For this review, take the finished solid that the model builds, in its own axes (mm). Face numbers are marked on the shaded views. A direction names the side the tool comes from. Give positions to 0.01 mm unless a question says otherwise; leave off trailing zeros. Write each loop counter-clockwise with the first axis right and the second up, starting at its lowest first coordinate (ties: lowest second). Pieces come first, ordered by that corner, then holes. Notation, with made-up numbers: M 59.25,-25.5 L 112.25,-25.5 A23 cw 112.25,8.5 Z; hole C 45,-13 d7. An arc over 180 degrees is marked long. Write item = value, one per line.
```python
from build123d import *

# Parameters (mm, degrees)
F1_DEPTH = 8
F2_R     = 3
F3_DEPTH = 8
F4_R     = 4
F5_DEPTH = 8
F6_W     = 9
F6_H     = 2
F7_DEPTH = 3


with BuildPart() as f1:
    # F0 (on Top) → F1 (new body)
    with BuildSketch(Plane.XY):
        with BuildLine():
            Line((7, 20), (-7, 20))
            ThreePointArc((-7, 20), (-9.12132, 19.12132), (-10, 17))
            Line((-10, 17), (-10, -17))
            ThreePointArc((-10, -17), (-9.12132, -19.12132), (-7, -20))
            Line((-7, -20), (7, -20))
            ThreePointArc((7, -20), (9.12132, -19.12132), (10, -17))
            Line((10, -17), (10, 17))
            ThreePointArc((10, 17), (9.12132, 19.12132), (7, 20))
        make_face()
    extrude(amount=F1_DEPTH)

    # F2 (on face) → F3 (cut, through all)
    with BuildSketch(Plane.XY.offset(8)):
        with Locations((0, 12)):
            Circle(F2_R)
        with Locations((0, -12)):
            Circle(F2_R)
    extrude(amount=-F3_DEPTH, mode=Mode.SUBTRACT)

    # F4 (on face) → F5 (cut, through all)
    with BuildSketch(Plane.XY.offset(8)):
        Circle(F4_R)
    extrude(amount=-F5_DEPTH, mode=Mode.SUBTRACT)

    # F6 (on face) → F7 (join)
    with BuildSketch(Plane.XY.offset(8)):
        with Locations((0, -6.5)):
            Rectangle(F6_W, F6_H)
        with Locations((0, 6.5)):
            Rectangle(F6_W, F6_H)
    extrude(amount=F7_DEPTH)


solid = f1.part
```
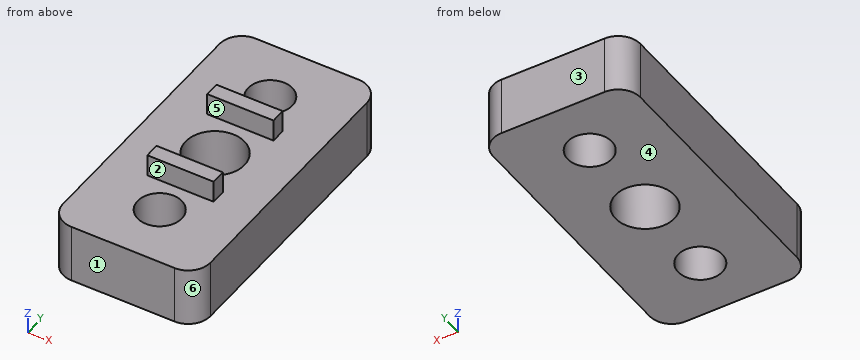
1. The part is to be moulded in two halves that separate along Y. For the marked faces 3, 4, 5 and 6, say which applies: +Y half, -Y half, draft (parallel to the pull), parting line (faces both ways), or undercut.
Responses:
face_3 = +Y half
face_4 = draft
face_5 = undercut
face_6 = -Y half
2. For line 1 along Y through (x, z) = (0, 5); line 2 along Y through (x, z) = (2.5, 4.5); line 3 along Z through (x, y) = (7, -4), list the stretches that pass through material, from the lowest coordinate up. Write a range as from..to.
Responses:
line_1 = -20..-15, -9..-4, 4..9, 15..20
line_2 = -20..-13.66, -10.34..-3.12, 3.12..10.34, 13.66..20
line_3 = 0..8
3. Machinability: for the marked faces 1 and 2, which of the approach directions +Z, -Z, +X, -X, +Y, -Y give a long, thin tool a straight path to every point of the face, cutting with its end or side? Answer none if there is none.
Responses:
face_1 = +Z, -Z, +X, -X, -Y
face_2 = +Z, +X, -X, -Y
4. Insertion check: P1, Ø1.6, axis at y = -6.5, z = 9, coming from the -X side; P2, Ø2.5, axis at x = -1.5, z = 10, coming from the -Y side; P3, Ø5, axis at x = 7, y = 1.5, coming from the +Z side. Each pin has a flat end and moves straight along its axis. Give the tip position at first contact, or say it passes through.
Responses:
P1 = -4.5
P2 = -7.5
P3 = 8
5. We need section C-C, the plane x = 0. Write out the cut boundary in (y, z).
Responses:
outline = M -20,0 L -15,0 L -15,8 L -20,8 Z; M -9,0 L -4,0 L -4,8 L -5.5,8 L -5.5,11 L -7.5,11 L -7.5,8 L -9,8 Z; M 4,0 L 9,0 L 9,8 L 7.5,8 L 7.5,11 L 5.5,11 L 5.5,8 L 4,8 Z; M 15,0 L 20,0 L 20,8 L 15,8 Z
6. We need section D-D, the plane z = 4. Write out the cut boundary in (x, y).
Responses:
outline = M -10,-17 A3 ccw -7,-20 L 7,-20 A3 ccw 10,-17 L 10,17 A3 ccw 7,20 L -7,20 A3 ccw -10,17 Z; hole C 0,0 d8; hole C 0,-12 d6; hole C 0,12 d6
7. We need section B-B, the plane z = 8.5. Write out the cut boundary in (x, y).
Responses:
outline = M -4.5,-7.5 L 4.5,-7.5 L 4.5,-5.5 L -4.5,-5.5 Z; M -4.5,5.5 L 4.5,5.5 L 4.5,7.5 L -4.5,7.5 Z
8. We need section A-A, the plane y = 0. Write out the cut boundary in (x, z).
Responses:
outline = M -10,0 L -4,0 L -4,8 L -10,8 Z; M 4,0 L 10,0 L 10,8 L 4,8 Z
